Can you work these out from the model? Positions are in its coordinate system, mm. A direction names the side the tool comes from. Coordinates: 2 decimals unless noted, no trailing zeros. Order: outer loops, then holes, each group sorted by start corner. A loop starts at its lowest first (then second) coordinate and runs counter-clockwise, first axis right, second up. Notation, with made-up numbers: (28.25, -18) -> (65.25, -18) arc R22 ccw to (65.25, 8) -> close; hole circle Ø3 at (21.25, -39.75). An arc over 180 degrees is marked (long way). Write item = value, one per line. Start each with the question number.
Autodesk Inventor part; units mm, degrees
ref_plane "Work Plane1" through (0, 0, 2.5) normal (0, 0, 1) x (1, 0, 0)
ref_plane "YZ Plane" through (0, 0, 0) normal (1, 0, 0) x (0, 1, 0)
ref_plane "XZ Plane" through (0, 0, 0) normal (0, 1, 0) x (-1, 0, 0)
sketch "Sketch1" plane through (0, 0, 0) normal (0, 0, 1) x (1, 0, 0)
  circle A0 centre (0, 0) radius 1.5
  circle A1 centre (0, 0) radius 4.5
  dimension "d0" = 3
  dimension "d1" = 9
extrude "Extrusion1" add sketch "Sketch1" along normal blind 5
sketch "Sketch2" plane through (0, 0, 5) normal (0, 0, 1) x (1, 0, 0)
  circle A0 centre (0, 0) radius 4.5
  circle A1 centre (0, 0) radius 1.5
  circle A2 centre (0, 0) radius 2
  circle A3 centre (0, 0) radius 4
  dimension "d4" = 0.5
  dimension "d5" = 0.5
extrude "Extrusion2" cut sketch "Sketch2" against normal blind 0.5 contours A3
ref_plane "Work Plane1" through (0, 0, 2.5) normal (0, 0, 1) x (1, 0, 0)
mirror "Mirror1" about plane through (0, 0, 2.5) normal (0, 0, 1) of "Extrusion2"
properties part number "603ZZ Roller Bearing"
(1) If I drill on L1, parallel to Y at x = 0, z = 0.3; L2, parallel to Z at x = 2, y = 2.75; L3, parallel to X at y = -0.5, z = 3.55, over which ranges is the centre line in solid material (lowest first)? Write a range as from..to.
(2) Imagine slicing it at D-D (x = 3.25). Write out the boundary of the cut face in (y, z).
(3) Thinking about a two-plate mould opening in X: for faces 4 (the face through (-0.867, 3.905, 0.246)), 5 (the face through (-0.59, -4.46, 2.46)), 6 (the face through (-3, -3, 0)), which applies, +X half, -X half, draft (parallel to the pull), parting line (faces both ways), or undercut?
(4) Imagine slicing it at A-A (y = 0). Write out the boundary of the cut face in (x, z).
(5) For faces 1 (the face through (-1.5, -0.07, 2.46)), 2 (the face through (-0.434, 1.952, 0.246)), 3 (the face through (-0.434, -1.952, 4.754)), which set-ups out of +Z, -Z, +X, -X, +Y, -Y let a thin tool reach every point of the face, with its end or its side?
(6) Imagine slicing it at C-C (z = 2.15). Write out the boundary of the cut face in (x, y), plus the area to 3 significant figures.
Result set:
q1.L1 = -4.5..-4, -2..-1.5, 1.5..2, 4..4.5
q1.L2 = 0.5..4.5
q1.L3 = -4.47..-1.41, 1.41..4.47
q2.outline = (-3.11, 0) -> (-2.33, 0) -> (-2.33, 0.5) -> (2.33, 0.5) -> (2.33, 0) -> (3.11, 0) -> (3.11, 5) -> (2.33, 5) -> (2.33, 4.5) -> (-2.33, 4.5) -> (-2.33, 5) -> (-3.11, 5) -> close
q3.face_4 = undercut
q3.face_5 = parting line
q3.face_6 = draft
q4.outline = (-4.5, 0) -> (-4, 0) -> (-4, 0.5) -> (-2, 0.5) -> (-2, 0) -> (-1.5, 0) -> (-1.5, 5) -> (-2, 5) -> (-2, 4.5) -> (-4, 4.5) -> (-4, 5) -> (-4.5, 5) -> close; (1.5, 0) -> (2, 0) -> (2, 0.5) -> (4, 0.5) -> (4, 0) -> (4.5, 0) -> (4.5, 5) -> (4, 5) -> (4, 4.5) -> (2, 4.5) -> (2, 5) -> (1.5, 5) -> close
q5.face_1 = +Z, -Z
q5.face_2 = -Z
q5.face_3 = +Z
q6.outline = circle Ø9 at (0, 0); hole circle Ø3 at (0, 0)
q6.area = 56.5 mm2
